from build123d import *

# Parameters (mm, degrees)
SKETCH_1_W      = 12
SKETCH_1_H      = 8
EXTRUDE_1_DEPTH = 7
EXTRUDE_2_DEPTH = 7
EXTRUDE_5_DEPTH = 7
EXTRUDE_START   = -1
EXTRUDE_6_DEPTH = 5


with BuildPart() as part:
    # 草图1 → 凸台-拉伸1 (new body)
    with BuildSketch(Plane(origin=(0, 0, 0), x_dir=(1, 0, 0), z_dir=(0, 1, 0))):
        with Locations((6, 4)):
            Rectangle(SKETCH_1_W, SKETCH_1_H)
    extrude(amount=EXTRUDE_1_DEPTH)

    # 草图2 → 凸台-拉伸2 (add)
    with BuildSketch(Plane(origin=(0, 7, 0), x_dir=(1, 0, 0), z_dir=(0, 1, 0))):
        Polygon((-3, -1.45), (0, -1.45), (0, 0), (0, 4), (-3, 4), align=None)
        Polygon((-3, 9.45), (-3, 4), (0, 4), (0, 8), (0, 9.45), align=None)
    extrude(amount=-EXTRUDE_2_DEPTH)

    # 草图3 → 凸台-拉伸5 (add)
    with BuildSketch(Plane(origin=(0, 7, 0), x_dir=(1, 0, 0), z_dir=(0, 1, 0))):
        Polygon((-3.384615385, 4), (-3, 4.5), (-8, 11), (-8, 10), align=None)
        Polygon((-3, 3.5), (-3.384615385, 4), (-8, -2), (-8, -3), align=None)
        Polygon((-3, 3.5), (-3, 4.5), (-3.384615385, 4), align=None)
    extrude(amount=-EXTRUDE_5_DEPTH)

    # 草图4 → 凸台-拉伸6 (add)
    with BuildSketch(Plane(origin=(0, 7, 0), x_dir=(1, 0, 0), z_dir=(0, 1, 0)).offset(EXTRUDE_START)):
        Polygon((2, 8), (2, 8.65), (3, 8), align=None)
        Polygon((2, 0), (2, -0.65), (4.058075402, 0), align=None)
    extrude(amount=-EXTRUDE_6_DEPTH)


solid = part.part
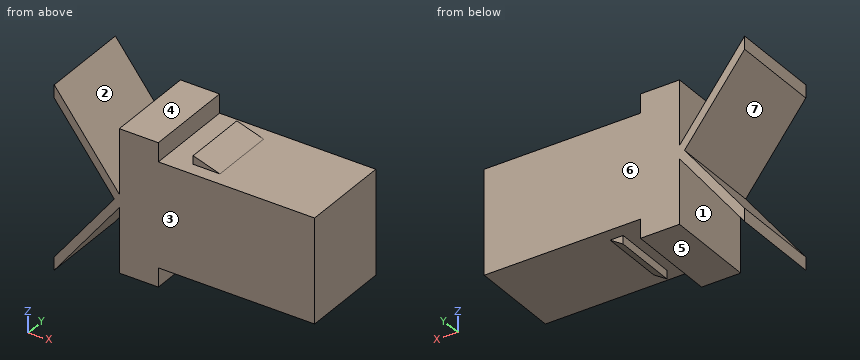
Model file for the job. Use its own axes, mm. Face numbers are marked on the shaded views. A direction names the side the tool comes from. Round coordinates to 2 decimals unless told otherwise and drop trailing zeros. Loops run counter-clockwise (first coordinate to the right, second up) from the corner with the lowest first, then second, coordinate; pieces in that order, holes last.
1. Mould opens along Z. For the marked faces 4, 5, 6 and 7 say: +Z half, -Z half, draft (parallel to the pull), parting line (faces both ways), or undercut.
Check values:
face 4: +Z half
face 5: -Z half
face 6: draft
face 7: undercut
2. Band-saw the part on C-C, the plane x = 8. List the corners of the cut face in (y, z), and give its area (3 significant figures).
Check values:
outline: (0, -8) - (7, -8) - (7, 0) - (0, 0) - close
area: 56.0 mm2
3. Wall check: probe 1 along Z at (x, y) = (-0.5, 6.5); probe 2 along Z at (x, y) = (5.5, 5.75); probe 3 along Z at (x, y) = (-3.5, 3.5). Give the ranges that are in metal, low to high.
Check values:
probe 1: z = -9.45 to 1.45
probe 2: z = -8 to 0
probe 3: z = -5.15 to -4.15, -3.85 to -2.85
4. Drop flat-ended pins along their axis: P1, Ø2, axis at x = -3, y = 5, coming from the -Z side; P2, Ø0.5, axis at x = 2.5, z = -8.5, coming from the +Y side; P3, Ø2, axis at x = 5.5, y = 4, coming from the -Z side. Give the stop position or say it passes through.
Check values:
P1: stops at z = -9.45
P2: stops at y = 6
P3: stops at z = -8
5. Tool access for the marked faces 1, 2 and 3: list every direction of +Z, -Z, +X, -X, +Y, -Y with a clear straight run to the whole face (end or side of a thin tool).
Check values:
face 1: -Z, +Y, -Y
face 2: +Z, +Y, -Y
face 3: +Z, -Z, +X, -X, -Y
6. Band-saw the part on D-D, the plane z = -9.75. List the corners of the cut face in (x, y).
Check values:
outline: (-7.81, 0) - (-7.04, 0) - (-7.04, 7) - (-7.81, 7) - close
7. Band-saw the part on A-A, the plane z = -1.25. List the corners of the cut face in (x, y), and give its area (3 significant figures).
Check values:
outline: (-5.5, 0) - (-4.73, 0) - (-4.73, 7) - (-5.5, 7) - close; (-3, 0) - (12, 0) - (12, 7) - (-3, 7) - close
area: 110 mm2
8. Band-saw the part on B-B, the plane y = 2.75. List the corners of the cut face in (x, z), and give its area (3 significant figures).
Check values:
outline: (-8, -11) - (-3, -4.5) - (-3, -9.45) - (0, -9.45) - (0, -8) - (2, -8) - (2, -8.65) - (3, -8) - (12, -8) - (12, 0) - (4.06, 0) - (2, 0.65) - (2, 0) - (0, 0) - (0, 1.45) - (-3, 1.45) - (-3, -3.5) - (-8, 3) - (-8, 2) - (-3.38, -4) - (-8, -10) - close
area: 140 mm2
